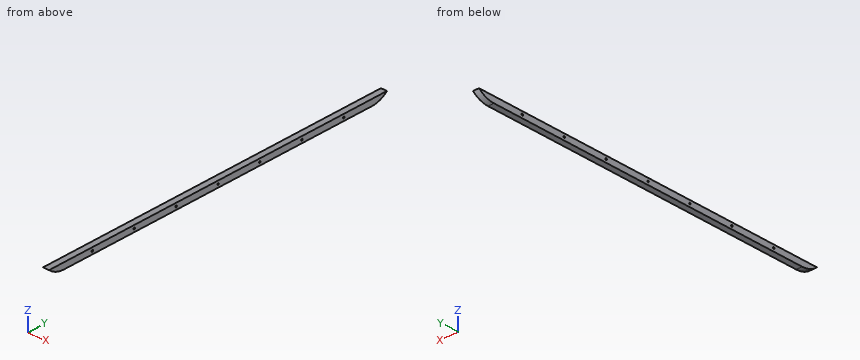
from build123d import *

# Parameters (mm, degrees)
F0_W        = 6.35
F0_H        = 6.35
F1_DEPTH    = 190.5
F2_T1_DEPTH = 90.3526041263
F4_D        = 1.778


# Not quite as in the source:
# - a fillet or chamfer that OpenCascade refuses, or shapes differently, is made with other operations: its cross-section is extruded or revolved along the edge and cut away or added


with BuildPart() as f1:
    # F0 (on Front) → F1 (new body, symmetric)
    with BuildSketch(Plane.XZ):
        Rectangle(F0_W, F0_H)
    extrude(amount=F1_DEPTH, both=True)

    # F2: fillet of radius 25.4 on 2 edges, made by hand

    # F2_s2 → F2_t1 (cut)
    with BuildSketch(Plane.YZ.offset(-45.1763020632)):
        with BuildLine():
            ThreePointArc((-173.6994791747, -3.175), (-182.6797352958, -1.534524406), (-190.5, 3.175))
            Line((-190.5, 3.175), (-190.5, -3.175))
            Line((-190.5, -3.175), (-173.6994791747, -3.175))
        make_face()
        with BuildLine():
            ThreePointArc((173.6994791747, -3.175), (182.6797352958, -1.534524406), (190.5, 3.175))
            Line((190.5, 3.175), (190.5, -3.175))
            Line((190.5, -3.175), (173.6994791747, -3.175))
        make_face()
    extrude(amount=F2_T1_DEPTH, mode=Mode.SUBTRACT)

    # F4 (through all)
    with Locations(Plane.YZ.offset(3.175)):
        with Locations((47.244, 0), (94.488, 0), (141.732, 0), (0, 0), (-47.244, 0), (-94.488, 0), (-141.732, 0)):
            Hole(F4_D / 2)


solid = f1.part
Source: CAD feature listing. Evaluate the final solid. Frame: model axes, mm. Coordinates: 2 decimals unless noted, no trailing zeros. Loops run counter-clockwise (first coordinate to the right, second up) from the corner with the lowest first, then second, coordinate; pieces in that order, holes last. Notation, with made-up numbers: M 53.5,-0.75 L 82.5,-0.75 A9 cw 82.5,5.25 Z; hole C 83.5,-27 d3. An arc over 180 degrees is marked long. Answer in a Markdown table with one row per item.
Q1. Section A-A on x = 1.25. Return the cut outline in (y, z) (3 decimals).
Answers below:
| item | result |
|---|---|
| outline | M -190.5,3.175 A25.4 ccw -173.699,-3.175 L 173.699,-3.175 A25.4 ccw 190.5,3.175 Z; hole C -141.732,0 d1.778; hole C -94.488,0 d1.778; hole C -47.244,0 d1.778; hole C 0,0 d1.778; hole C 47.244,0 d1.778; hole C 94.488,0 d1.778; hole C 141.732,0 d1.778 |
Q2. Ray query, probe 1 along Z at (x, y) = (1.25, 0) (3 decimals); probe 2 along Y at (x, z) = (2.75, 1.5); probe 3 along Y at (x, z) = (-1, 1.25). Return the intervals inside material, ascending. Write a range as from..to.
Answers below:
| item | result |
|---|---|
| probe 1 | z = -3.175..-0.889, 0.889..3.175 |
| probe 2 | y = -188.38..188.38 |
| probe 3 | y = -188.02..188.02 |
Q3. First-contact query: pin 1 (2 mm diameter, centred on x = 0, z = 1.5, fed in from -Y). Flat tip, straight axial feed; report the tip coordinate or a pass-through.
Answers below:
| item | result |
|---|---|
| pin 1 | stops at y = -189.7 |
